from build123d import *

# Parameters (mm, degrees)
SKETCH1_W           = 225.11
SKETCH1_H           = 188
BOSS_EXTRUDE1_DEPTH = 5
SKETCH2_R           = 2
CUT_EXTRUDE1_DEPTH  = 10
SKETCH3_W           = 40
SKETCH3_H           = 5
BOSS_EXTRUDE2_DEPTH = 5
SKETCH5_W           = 5
SKETCH5_H           = 40
SKETCH5_W_2         = 40
SKETCH5_H_2         = 5
BOSS_EXTRUDE3_DEPTH = 5
CUT_EXTRUDE2_DEPTH  = 5
CUT_EXTRUDE3_DEPTH  = 5
SKETCH8_W           = 30
SKETCH8_H           = 5
CUT_EXTRUDE4_DEPTH  = 5
SKETCH9_W           = 30.000010782
SKETCH9_H           = 5
CUT_EXTRUDE5_DEPTH  = 5
CUT_EXTRUDE6_DEPTH  = 15
BOSS_EXTRUDE4_DEPTH = 5


with BuildPart() as part:
    # Sketch1 → Boss-Extrude1 (new body)
    with BuildSketch(Plane.XY):
        Rectangle(SKETCH1_W, SKETCH1_H)
    extrude(amount=BOSS_EXTRUDE1_DEPTH)

    # Sketch2 → Cut-Extrude1 (cut)
    with BuildSketch(Plane.XY.offset(5)):
        with Locations((-19.714505863, -13)):
            Circle(SKETCH2_R)
        with Locations((-4.214505863, -13)):
            Circle(SKETCH2_R)
        with Locations((-4.214505863, -27)):
            Circle(SKETCH2_R)
        with Locations((-19.714505863, -27)):
            Circle(SKETCH2_R)
    extrude(amount=-CUT_EXTRUDE1_DEPTH, mode=Mode.SUBTRACT)

    # Sketch3 → Boss-Extrude2 (add)
    with BuildSketch(Plane.XZ.offset(94)):
        with Locations((-52.555, 2.5)):
            Rectangle(SKETCH3_W, SKETCH3_H)
        with Locations((52.555, 2.5)):
            Rectangle(SKETCH3_W, SKETCH3_H)
    extrude(amount=BOSS_EXTRUDE2_DEPTH)

    # Sketch5 → Boss-Extrude3 (add)
    with BuildSketch(Plane.XY.offset(5)):
        with Locations((115.055, -44)):
            Rectangle(SKETCH5_W, SKETCH5_H)
        with Locations((115.041030137, 44)):
            Rectangle(SKETCH5_W, SKETCH5_H)
        with Locations((52.555, 96.5)):
            Rectangle(SKETCH5_W_2, SKETCH5_H_2)
        with Locations((-52.555, 96.5)):
            Rectangle(SKETCH5_W_2, SKETCH5_H_2)
        with Locations((-115.041030137, 44)):
            Rectangle(SKETCH5_W, SKETCH5_H)
        with Locations((-115.055, -44)):
            Rectangle(SKETCH5_W, SKETCH5_H)
    extrude(amount=-BOSS_EXTRUDE3_DEPTH)

    # Sketch6 → Cut-Extrude2 (cut)
    with BuildSketch(Plane.XY.offset(5)):
        Polygon((112.555, -2.1), (107.555, -2.1), (107.555, -5), (97.555, -5), (97.555, 5), (107.555, 5), (107.555, 2.1), (112.555, 2.1), align=None)
        Polygon((2.1, -94), (2.1, -89), (5, -89), (5, -79), (-5, -79), (-5, -89), (-2.1, -89), (-2.1, -94), align=None)
        Polygon((-2.1, 94), (-2.1, 89), (-5, 89), (-5, 79), (5, 79), (5, 89), (2.1, 89), (2.1, 94), align=None)
        Polygon((-112.555, 2.1), (-107.555, 2.1), (-107.555, 5), (-97.555, 5), (-97.555, -5), (-107.555, -5), (-107.555, -2.1), (-112.555, -2.1), align=None)
    extrude(amount=-CUT_EXTRUDE2_DEPTH, mode=Mode.SUBTRACT)

    # Sketch7 → Cut-Extrude3 (cut)
    with BuildSketch(Plane.XY.offset(5)):
        with BuildLine():
            Line((12.585494137, -53), (-37.414505863, -53))
            ThreePointArc((-37.414505863, -53), (-40.950039769, -51.535533906), (-42.414505863, -48))
            Line((-42.414505863, -48), (-42.414505863, -43))
            ThreePointArc((-42.414505863, -43), (-40.950039769, -39.464466094), (-37.414505863, -38))
            Line((-37.414505863, -38), (12.585494137, -38))
            ThreePointArc((12.585494137, -38), (16.121028043, -39.464466094), (17.585494137, -43))
            Line((17.585494137, -43), (17.585494137, -48))
            ThreePointArc((17.585494137, -48), (16.121028043, -51.535533906), (12.585494137, -53))
        make_face()
    extrude(amount=-CUT_EXTRUDE3_DEPTH, mode=Mode.SUBTRACT)

    # Sketch8 → Cut-Extrude4 (cut)
    with BuildSketch(Plane.XY.offset(5)):
        with Locations((71.270247069, -23.5)):
            Rectangle(SKETCH8_W, SKETCH8_H)
        with Locations((-71.299246748, -23.5)):
            Rectangle(SKETCH8_W, SKETCH8_H)
    extrude(amount=-CUT_EXTRUDE4_DEPTH, mode=Mode.SUBTRACT)

    # Sketch9 → Cut-Extrude5 (cut)
    with BuildSketch(Plane(origin=(0, 0, 0), x_dir=(-1, 0, 0), z_dir=(0, 0, -1))):
        with Locations((76.984802428, 58.5)):
            Rectangle(SKETCH9_W, SKETCH9_H)
        with Locations((-76.984802428, 58.5)):
            Rectangle(SKETCH9_W, SKETCH9_H)
    extrude(amount=-CUT_EXTRUDE5_DEPTH, mode=Mode.SUBTRACT)

    # Sketch10 → Cut-Extrude6 (cut)
    with BuildSketch(Plane.XY.offset(5)):
        with BuildLine():
            Line((92.555, -68), (42.555, -68))
            ThreePointArc((42.555, -68), (34.555, -60), (42.555, -52))
            Line((42.555, -52), (92.555, -52))
            ThreePointArc((92.555, -52), (100.555, -60), (92.555, -68))
        make_face()
        with BuildLine():
            Line((92.555, 10.043404022), (42.555, 10.043404022))
            ThreePointArc((42.555, 10.043404022), (34.555, 18.043404022), (42.555, 26.043404022))
            Line((42.555, 26.043404022), (92.555, 26.043404022))
            ThreePointArc((92.555, 26.043404022), (100.555, 18.043404022), (92.555, 10.043404022))
        make_face()
        with BuildLine():
            Line((-92.555, 10.043404022), (-42.555, 10.043404022))
            ThreePointArc((-42.555, 10.043404022), (-34.555, 18.043404022), (-42.555, 26.043404022))
            Line((-42.555, 26.043404022), (-92.555, 26.043404022))
            ThreePointArc((-92.555, 26.043404022), (-100.555, 18.043404022), (-92.555, 10.043404022))
        make_face()
        with BuildLine():
            Line((-92.555, -68), (-42.555, -68))
            ThreePointArc((-42.555, -68), (-34.555, -60), (-42.555, -52))
            Line((-42.555, -52), (-92.555, -52))
            ThreePointArc((-92.555, -52), (-100.555, -60), (-92.555, -68))
        make_face()
    extrude(amount=-CUT_EXTRUDE6_DEPTH, mode=Mode.SUBTRACT)

    # Sketch11 → Boss-Extrude4 (add)
    with BuildSketch(Plane.XY.offset(5)):
        with BuildLine():
            Line((-92.555, -68), (-42.555, -68))
            ThreePointArc((-42.555, -68), (-34.555, -60), (-42.555, -52))
            Line((-42.555, -52), (-92.555, -52))
            ThreePointArc((-92.555, -52), (-100.555, -60), (-92.555, -68))
        make_face()
    extrude(amount=-BOSS_EXTRUDE4_DEPTH)


solid = part.part
Work out the finished part from the listing and answer in its coordinate system (mm). A direction names the side the tool comes from. Coordinates: 2 decimals unless noted, no trailing zeros. Write each loop counter-clockwise with the first axis right and the second up, starting at its lowest first coordinate (ties: lowest second). Pieces come first, ordered by that corner, then holes.
1. For faces 4 (the flat face through (-115, -24, 3)), 5 (the flat face through (72.555, 96, 3)), 6 (the flat face through (32.555, 96, 3)), 7 (the flat face through (-103, 5, 3)), 8 (the flat face through (-72.555, 96, 3)), determine the directions among +Z, -Z, +X, -X, +Y, -Y from which every point of the face is accessible in a straight line to the end or side of a thin tool.
Results list:
face 4: +Z, -Z, -X
face 5: +Z, -Z, +X, +Y
face 6: +Z, -Z, +Y
face 7: +Z, -Z
face 8: +Z, -Z, -X, +Y
2. The part is cut by section A-A, the plane y = -60. Write down the section's boundary in (x, z) (3 decimals).
Results list:
outline: (-117.555, 0) - (34.555, 0) - (34.555, 5) - (-117.555, 5) - close; (100.555, 0) - (117.555, 0) - (117.555, 5) - (100.555, 5) - close
3. For a pull along Y with two mould halves and no side action, classify faces 1 (the flat face through (-32.555, -96, 2)), 2 (the flat face through (68, -68, 3)), 3 (the flat face through (115, -64, 3)) as +Y half, -Y half, draft (parallel to the pull), parting line (faces both ways), or undercut.
Results list:
face 1: draft
face 2: undercut
face 3: -Y half
4. The part is cut by section C-C, the plane x = 77. Write down the section's boundary in (y, z), and give its area (3 significant figures).
Results list:
outline: (-94, 0) - (-68, 0) - (-68, 5) - (-94, 5) - close; (-52, 0) - (-26, 0) - (-26, 5) - (-52, 5) - close; (-21, 0) - (10.04, 0) - (10.04, 5) - (-21, 5) - close; (26.04, 0) - (56, 0) - (56, 5) - (26.04, 5) - close; (61, 0) - (94, 0) - (94, 5) - (61, 5) - close
area: 730 mm2
5. Flat-ended cylindrical pins translate along their axes: pin 1 (1 mm diameter, centred on x = 12.5, z = 2.5, fed in from -Y); pin 2 (3 mm diameter, centred on y = 3, z = 1.5, fed in from +X) (3 decimals); pin 3 (3 mm diameter, centred on y = 61, z = 1, fed in from -X). Find the tip coordinate at first contact, or state that the pin passes through.
Results list:
pin 1: stops at y = -94
pin 2: stops at x = 112.555
pin 3: stops at x = -117.54
6. The part is cut by section D-D, the plane z = 3.1. State how many separate pieces and enclosed holes the cut face has, and give its area (3 significant figures).
Results list:
separate pieces: 1
enclosed holes: 12
area: 38,900 mm2
7. Consider line 1 along Y through (x, z) = (-81.5, 3.15); line 2 along Y through (x, z) = (-20, 3.85); line 3 along Y through (x, z) = (75, 4.35). Determine where each line is inside the solid, lowest interval first.
Results list:
line 1: y = -94 to -26, -21 to 10.04, 26.04 to 56, 61 to 94
line 2: y = -94 to -53, -38 to -28.98, -25.02 to -14.98, -11.02 to 94
line 3: y = -94 to -68, -52 to -26, -21 to 10.04, 26.04 to 56, 61 to 94
8. The part is cut by section B-B, the plane x = -53. Write down the section's boundary in (y, z).
Results list:
outline: (-99, 0) - (10.04, 0) - (10.04, 5) - (-99, 5) - close; (26.04, 0) - (99, 0) - (99, 5) - (26.04, 5) - close
